from build123d import *

# Parameters (mm, degrees)
F0_W           = 14
F0_H           = 14
F0_W_2         = 11.6
F0_H_2         = 4
F1_DEPTH       = 1.5
F2_D           = 5.3086
F2_CSINK_D     = 6.477
F2_CSINK_ANGLE = 82
F3_R           = 1.27


with BuildPart() as f1:
    # F0 (on Top) → F1 (new body)
    with BuildSketch(Plane.XY):
        with BuildLine():
            ThreePointArc((0, 2.54), (0.7439487758, 0.7439487758), (2.54, 0))
            Line((2.54, 0), (108.585, 0))
            ThreePointArc((108.585, 0), (110.3810512242, 0.7439487758), (111.125, 2.54))
            Line((111.125, 2.54), (111.125, 51.435))
            ThreePointArc((111.125, 51.435), (110.3810512242, 53.2310512242), (108.585, 53.975))
            Line((108.585, 53.975), (2.54, 53.975))
            ThreePointArc((2.54, 53.975), (0.7439487758, 53.2310512242), (0, 51.435))
            Line((0, 51.435), (0, 2.54))
        make_face()
        with Locations((17.4117, 17.4475)):
            Rectangle(F0_W, F0_H, mode=Mode.SUBTRACT)
        with Locations((36.4871, 17.4475)):
            Rectangle(F0_W, F0_H, mode=Mode.SUBTRACT)
        with Locations((55.5625, 17.4475)):
            Rectangle(F0_W, F0_H, mode=Mode.SUBTRACT)
        with Locations((74.6379, 17.4475)):
            Rectangle(F0_W, F0_H, mode=Mode.SUBTRACT)
        with Locations((93.7133, 17.4475)):
            Rectangle(F0_W, F0_H, mode=Mode.SUBTRACT)
        with Locations((17.4117, 36.5229)):
            Rectangle(F0_W_2, F0_H_2, mode=Mode.SUBTRACT)
        with Locations((36.4871, 36.5229)):
            Rectangle(F0_W, F0_H, mode=Mode.SUBTRACT)
        with Locations((55.5625, 36.5229)):
            Rectangle(F0_W, F0_H, mode=Mode.SUBTRACT)
        with Locations((74.6379, 36.5229)):
            Rectangle(F0_W, F0_H, mode=Mode.SUBTRACT)
        with Locations((93.7133, 36.5229)):
            Rectangle(F0_W, F0_H, mode=Mode.SUBTRACT)
    extrude(amount=-F1_DEPTH)

    # F2 (through all)
    with Locations(Plane.XY):
        with Locations((5.08, 48.895), (5.08, 5.08), (106.045, 5.08), (106.045, 48.895)):
            CounterSinkHole(F2_D / 2, F2_CSINK_D / 2, counter_sink_angle=F2_CSINK_ANGLE)

    # F3
    f3_edges = [f1.edges().sort_by_distance(p)[0] for p in [
        (55.5625, 0, 0),
        (111.125, 26.9875, 0),
        (110.381051, 0.743949, 0),
        (110.381051, 53.231051, 0),
        (55.5625, 53.975, 0),
        (0.743949, 53.231051, 0),
        (0, 26.9875, 0),
        (0.743949, 0.743949, 0),
    ]]
    fillet(f3_edges, radius=F3_R)


solid = f1.part
Design review of the part built by this model. Coordinates are the model's own, in mm. Give positions to 0.01 mm unless a question says otherwise; leave off trailing zeros. Return JSON: item names as keys, results as strings. Group by question number.
Item 1: The part is to be moulded in two halves that separate along X. For faces 1 (the cylindrical face through (3.653, 7.318, -1.092)), 2 (the flat face through (55, 27, 0)), 3 (the cylindrical face through (103.513, 5.877, -1.092)), say which applies: pulls with the +X half, pulls with the -X half, needs draft (parallel to the pull), parting line crosses it, or undercut.
Item 2: Wall thickness on line 1 along Y through (x, z) = (68, -1.15); line 2 along Y through (x, z) = (5.08, -1.1); line 3 along X through (y, z) = (42, -1.1): over which ranges is each line inside the solid? List them lowest first.
Item 3: Take a section at A-A (y = 5.08). Count the separate pieces of the cut face and the enclosed holes in it, plus the area to 3 significant figures.
Return value:
{
 "1": {"face 1": "undercut", "face 2": "needs draft", "face 3": "undercut"},
 "2": {"line 1": "y = 0.01 to 10.45, 24.45 to 29.52, 43.52 to 53.97", "line 2": "y = 0.01 to 2.43, 7.73 to 46.24, 51.55 to 53.96", "line 3": "x = 0.01 to 29.49, 43.49 to 48.56, 62.56 to 67.64, 81.64 to 86.71, 100.71 to 111.11"},
 "3": {"separate pieces": "3", "enclosed holes": "0", "area": "149 mm2"}
}
